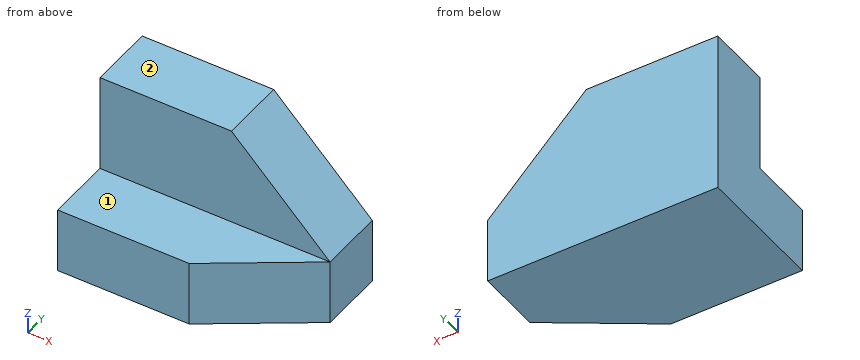
```python
from build123d import *

# Parameters (mm, degrees)
F0_W     = 44.45
F0_H     = 31.75
F1_DEPTH = 25.4
F2_W     = 44.45
F2_H     = 19.05
F3_DEPTH = 12.7
F5_DEPTH = 12.701
F7_DEPTH = 12.701


with BuildPart() as f1:
    # F0 (on Front) → F1 (new body)
    with BuildSketch(Plane.XZ):
        with Locations((22.225, 15.875)):
            Rectangle(F0_W, F0_H)
    extrude(amount=F1_DEPTH)

    # F2 (on face) → F3 (cut)
    with BuildSketch(Plane.XZ.offset(25.4)):
        with Locations((22.225, 22.225)):
            Rectangle(F2_W, F2_H)
    extrude(amount=-F3_DEPTH, mode=Mode.SUBTRACT)

    # F4 (on face) → F5 (cut, through all)
    with BuildSketch(Plane.XZ.offset(12.7)):
        Polygon((44.45, 31.75), (25.4, 31.75), (44.45, 12.7), align=None)
    extrude(amount=-F5_DEPTH, mode=Mode.SUBTRACT)

    # F6 (on face) → F7 (cut, through all)
    with BuildSketch(Plane.XY.offset(12.7)):
        Polygon((44.45, -25.4), (44.45, -12.7), (25.4, -25.4), align=None)
    extrude(amount=-F7_DEPTH, mode=Mode.SUBTRACT)


solid = f1.part
```
Could you check a few things on this model? Use its own coordinates, in mm. Face numbers are marked on the shaded views. A direction names the side the tool comes from. Give positions to 0.01 mm unless a question says otherwise; leave off trailing zeros. Order: outer loops, then holes, each group sorted by start corner. A loop starts at its lowest first (then second) coordinate and runs counter-clockwise, first axis right, second up.
Q1. Suppose I cut it at A-A, the plane z = 10.5. Write out the boundary of the cut face in (x, y), and give its area (3 significant figures).
Q2. If I drill on line 1 along Z through (x, y) = (30, -19); line 2 along Y through (x, z) = (29.5, 14); line 3 along Z through (x, y) = (28, -2.25), over which ranges is the centre line in solid material (lowest first)?
Q3. Suppose I cut it at D-D, the plane x = 3. Write out the boundary of the cut face in (y, z), and give its area (3 significant figures).
Q4. Suppose I cut it at B-B, the plane y = -6.75. Write out the boundary of the cut face in (x, z).
Q5. Suppose I cut it at C-C, the plane x = 36.5. Write out the boundary of the cut face in (y, z).
Q6. For the marked faces 1 and 2, which set-ups out of +Z, -Z, +X, -X, +Y, -Y let a thin tool reach every point of the face, with its end or its side?
Q7. I'm going to push flat-ended pins straight in: P1, Ø10, axis at y = -15, z = 24, coming from the -X side; P2, Ø10, axis at x = 22.5, z = 18.5, coming from the -Y side. Where does each tip first touch, or does it pass through?
Solution:
1. outline: (0, -25.4) - (25.4, -25.4) - (44.45, -12.7) - (44.45, 0) - (0, 0) - close
1. area: 1,010 mm2
2. line 1: z = 0 to 12.7
2. line 2: y = -12.7 to 0
2. line 3: z = 0 to 29.15
3. outline: (-25.4, 0) - (0, 0) - (0, 31.75) - (-12.7, 31.75) - (-12.7, 12.7) - (-25.4, 12.7) - close
3. area: 565 mm2
4. outline: (0, 0) - (44.45, 0) - (44.45, 12.7) - (25.4, 31.75) - (0, 31.75) - close
5. outline: (-18, 0) - (0, 0) - (0, 20.65) - (-12.7, 20.65) - (-12.7, 12.7) - (-18, 12.7) - close
6. face 1: +Z, +X, -X, -Y
6. face 2: +Z, +X, -X, +Y, -Y
7. P1: stops at x = 0
7. P2: stops at y = -12.7
